Verification items for the finished model (mm, model axes). Face numbers are marked on the shaded views. A direction names the side the tool comes from. Give positions to 0.01 mm unless a question says otherwise; leave off trailing zeros. Loops run counter-clockwise (first coordinate to the right, second up) from the corner with the lowest first, then second, coordinate; pieces in that order, holes last. Notation, with made-up numbers: M 68,33.25 L 88,33.25 A18 cw 88,45.25 Z; hole C 64.25,40 d7. An arc over 180 degrees is marked long. Answer in a Markdown table with one row per item.
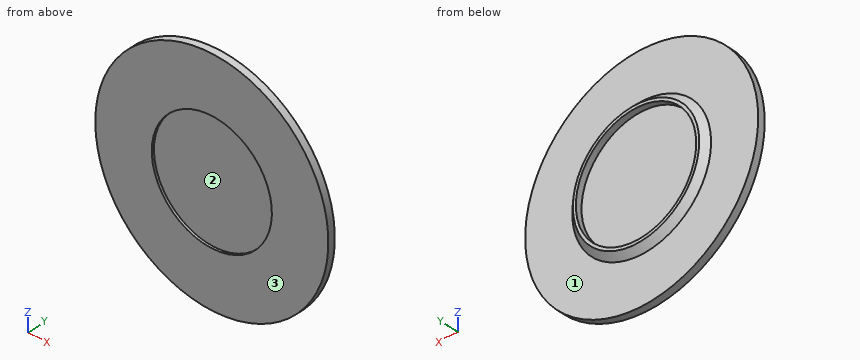
Autodesk Inventor part; units mm, degrees
ref_plane "YZ Plane" through (0, 0, 0) normal (1, 0, 0) x (0, 1, 0)
ref_plane "XZ Plane" through (0, 0, 0) normal (0, 1, 0) x (-1, 0, 0)
ref_plane "XY Plane" through (0, 0, 0) normal (0, 0, 1) x (1, 0, 0)
sketch "Эскиз1" plane through (0, 0, 0) normal (0, 1, 0) x (-1, 0, 0)
  circle A0 centre (0, 0) radius 25.05
  circle A1 centre (0, 0) radius 48.5
  circle A2 centre (0, 0) radius 26.3
  dimension "d1" = 50.1
  dimension "d2" = 97
  dimension "d3" = 52.6
extrude "Выдавливание1" add sketch "Эскиз1" against normal blind 3 contours A0 | A1 | A2
extrude "Выдавливание2" add sketch "Эскиз1" along normal blind 2.6 contours A2
sketch "Эскиз2" plane through (0, -3, 0) normal (0, -1, 0) x (1, 0, 0)
  point P0 (0, 0)
hole "Отверстие1" at (0, -3, 0) direction (0, 1, 0) diameter 50 depth 1
chamfer "Фаска1" distance 2.6 angle 45 1 edges at (26.3, 0, 0)
properties part number "навес над зеркалом"
Item 1: Tool access check on the marked faces 1, 2 and 3. Record the directions out of +Z, -Z, +X, -X, +Y, -Y that give a thin tool (end or side, any length) a straight path to the whole face; none if there is none.
Reported:
| item | result |
|---|---|
| face 1 | +Y |
| face 2 | -Y |
| face 3 | +Z, -Z, +X, -X, -Y |
Item 2: Sectioned sample at C-C (y = -0.9). Record the cut outline in (x, z).
Reported:
| item | result |
|---|---|
| outline | C 0,0 d97 |
Item 3: Scan lines: L1, parallel to Z at x = 0, y = -2.3; L2, parallel to Y at x = 43, z = -13.5; L3, parallel to Y at x = 13, z = 10. Record each from-to range of solid material in increasing order. Write a range as [from, to].
Reported:
| item | result |
|---|---|
| L1 | z = [-48.5, -25], [25, 48.5] |
| L2 | y = [-3, 0] |
| L3 | y = [-2, 0] |
Item 4: Go/stop test with flat-tipped pins: pin 1 (1.5 mm diameter, centred on x = 31, z = 37.5, fed in from -Y); pin 2 (1.5 mm diameter, centred on x = 37.5, z = 2.5, fed in from +Y); pin 3 (3 mm diameter, centred on y = -2, z = 9, fed in from -X); pin 4 (15 mm diameter, centred on x = 5, z = -2.5, fed in from -Y). Record where each tip stops, or that it passes through.
Reported:
| item | result |
|---|---|
| pin 1 | stops at y = -3 |
| pin 2 | stops at y = 0 |
| pin 3 | stops at x = -47.92 |
| pin 4 | stops at y = -2 |
Item 5: Sectioned sample at D-D (x = -34). Record the cut outline in (y, z), and give its area (3 significant figures).
Reported:
| item | result |
|---|---|
| outline | M -3,-34.59 L 0,-34.59 L 0,34.59 L -3,34.59 Z |
| area | 208 mm^2 |
